```python
from build123d import *

# Parameters (mm, degrees)
F1_DEPTH = 25.4


# Not quite as in the source:
# - a feature names something its author has since deleted; it is built from what else it names


with BuildPart() as f1:
    # F0 (on Front) → F1 (new body)
    with BuildSketch(Plane.XZ):
        with BuildLine():
            ThreePointArc((3.5129496086, 128.2487611501), (-124.8295958309, -0.0937842894), (3.5129496086, -128.4363297289))
            Line((3.5129496086, -128.4363297289), (187.7788752317, -128.4363297289))
            Line((187.7788752317, -128.4363297289), (187.7788752317, -156.6303297289))
            Line((187.7788752317, -156.6303297289), (230.9588752317, -156.6303297289))
            Line((230.9588752317, -156.6303297289), (230.9588752317, -128.4363297289))
            Line((230.9588752317, -128.4363297289), (230.9588752317, -100.2423297289))
            Line((230.9588752317, -100.2423297289), (3.5129496086, -100.2423297289))
            ThreePointArc((3.5129496086, -100.2423297289), (-96.5909865333, -0.138393587), (3.5129496086, 99.9655425549))
            Line((3.5129496086, 99.9655425549), (230.9588752317, 100.0547611501))
            Line((230.9588752317, 100.0547611501), (230.9588752317, 128.2487611501))
            Line((230.9588752317, 128.2487611501), (230.9588752317, 156.4427611501))
            Line((230.9588752317, 156.4427611501), (187.7788752317, 156.4427611501))
            Line((187.7788752317, 156.4427611501), (187.7788752317, 128.2487611501))
            Line((187.7788752317, 128.2487611501), (3.5129496086, 128.2487611501))
        make_face()
    extrude(amount=F1_DEPTH)


solid = f1.part
```
Source: CAD feature listing. Evaluate the final solid. Frame: model axes, mm. A direction names the side the tool comes from. Coordinates: 2 decimals unless noted, no trailing zeros. Order: outer loops, then holes, each group sorted by start corner. A loop starts at its lowest first (then second) coordinate and runs counter-clockwise, first axis right, second up. Notation, with made-up numbers: (73, -32) - (88, -32) arc R19 ccw to (88, -4) - close; hole circle Ø4 at (85, 35). An arc over 180 degrees is marked (long way). One line per item, written item: value.
1) Ray query, line 1 (Z direction, x = 118.5, y = -15); line 2 (Z direction, x = 214, y = -21.5); line 3 (X direction, y = -10, z = -140). Return the intervals inside material, ascending. Write a range as [from, to].
Computed values:
line 1: z = [-128.44, -100.24], [100.01, 128.25]
line 2: z = [-156.63, -100.24], [100.05, 156.44]
line 3: x = [187.78, 230.96]
2) Mould query, pull axis Z, two halves, no side actions, for faces 4 (the face through (-96.567, -12.522, -2.34)), 5 (the face through (65, -25.4, -104)), 6 (the face through (119, -13, -100.242)), 7 (the face through (94, -13, -128.436)). Classes: released by +Z, released by -Z, zero draft, split by the parting line, or undercut.
Computed values:
face 4: undercut
face 5: zero draft
face 6: undercut
face 7: released by -Z
3) Reachability of faces 1 (the face through (97, -13, 128.249)), 2 (the face through (230.959, -13, -129)), 3 (the face through (187.779, -13, -142)) from +Z, -Z, +X, -X, +Y, -Y: full face, straight path, thin tool, end or side. Return the list, or none.
Computed values:
face 1: +Z, -X, +Y, -Y
face 2: +Z, -Z, +X, +Y, -Y
face 3: -Z, -X, +Y, -Y
4) Cut plane A-A on x = 84. Output: boundary loops of the cut face in (y, z), plus the area to 3 significant figures.
Computed values:
outline: (-25.4, -128.44) - (0, -128.44) - (0, -100.24) - (-25.4, -100.24) - close; (-25.4, 100) - (0, 100) - (0, 128.25) - (-25.4, 128.25) - close
area: 1,430 mm^2
5) Cut plane D-D on z = -106. Output: boundary loops of the cut face in (x, y), plus the area to 3 significant figures.
Computed values:
outline: (-68.98, -25.4) - (230.96, -25.4) - (230.96, 0) - (-68.98, 0) - close
area: 7,620 mm^2
6) Cut plane B-B on y = -18.75. Output: boundary loops of the cut face in (x, z).
Computed values:
outline: (3.51, -128.44) - (187.78, -128.44) - (187.78, -156.63) - (230.96, -156.63) - (230.96, -100.24) - (3.51, -100.24) arc R100.1 cw to (3.51, 99.97) - (230.96, 100.05) - (230.96, 156.44) - (187.78, 156.44) - (187.78, 128.25) - (3.51, 128.25) arc R128.34 ccw to start
7) Cut plane C-C on x = -86. Output: boundary loops of the cut face in (y, z), plus the area to 3 significant figures.
Computed values:
outline: (-25.4, -92.07) - (0, -92.07) - (0, -44.95) - (-25.4, -44.95) - close; (-25.4, 44.67) - (0, 44.67) - (0, 91.88) - (-25.4, 91.88) - close
area: 2,400 mm^2
8) Contact query for flat-ended pins moving along their axis: pin 1 (1 mm diameter, centred on y = -19, z = -113, fed in from -X); pin 2 (3 mm diameter, centred on x = 62, y = -6, fed in from +Z); pin 3 (1 mm diameter, centred on y = -6.5, z = 90.5, fed in from +X). Output: stop coordinate, or through.
Computed values:
pin 1: stops at x = -58.43
pin 2: stops at z = 128.25
pin 3: stops at x = -37.89
